Can you work these out from the model? Positions are in its coordinate system, mm. Face numbers are marked on the shaded views. A direction names the side the tool comes from. Give positions to 0.01 mm unless a question says otherwise; leave off trailing zeros. Order: outer loops, then holes, each group sorted by start corner. A loop starts at its lowest first (then second) coordinate and runs counter-clockwise, first axis right, second up.
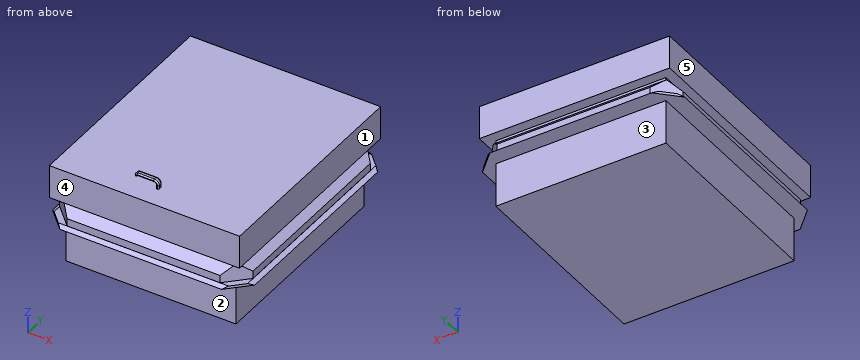
```python
from build123d import *

# Parameters (mm, degrees)
F0_W          = 675
F0_H          = 800
F1_DEPTH      = 270
F2_W          = 755
F2_H          = 880
F3_DEPTH      = 131.76
F5_START      = -175
F4_W          = 802
F4_H          = 926.8378600104
F5_DEPTH      = 10
F6_W          = 767
F6_H          = 892
F7_DEPTH      = 70
F8_SIZE       = 80
F9_SIZE       = 39.99999
F10_SIZE2     = 9.99999
F10_SIZE      = 16.99999
F13_W         = 10
F13_H         = 20
F15_R         = 3.5
F16_T1_DEPTH  = 65
F16_T3_DEPTH  = 3.5995793343
F16_T5_DEPTH  = 13.4709453487
F16_T8_ANGLE  = 90
F16_T10_ANGLE = 90
F16_T12_ANGLE = 90
F16_T14_ANGLE = 90
F16_T16_ANGLE = 90
F16_T18_ANGLE = 90
F16_T20_ANGLE = 90
F16_T22_ANGLE = 90


# Not quite as in the source:
# - a fillet or chamfer that OpenCascade refuses, or shapes differently, is made with other operations: its cross-section is extruded or revolved along the edge and cut away or added
# - a fillet or chamfer is up to 0.001 mm smaller than in the source, because OpenCascade refuses the exact size
# - a feature names something its author has since deleted; it is built from what else it names


with BuildPart() as f1:
    # F0 (on Top) → F1 (new body)
    with BuildSketch(Plane.XY):
        Rectangle(F0_W, F0_H)
    extrude(amount=F1_DEPTH)

    # F2 (on face) → F3 (join)
    with BuildSketch(Plane.XY.offset(270)):
        Rectangle(F2_W, F2_H)
    extrude(amount=F3_DEPTH)

    # F4 (on face) → F5 (join)
    with BuildSketch(Plane(origin=(0, 0, 0), x_dir=(1, 0, 0), z_dir=(0, 0, -1)).offset(F5_START)):
        Rectangle(F4_W, F4_H)
    extrude(amount=-F5_DEPTH)

    # F6 (on face) → F7 (join)
    with BuildSketch(Plane.XY.offset(185)):
        Rectangle(F6_W, F6_H)
    extrude(amount=F7_DEPTH)

    # F8
    f8_edges = [f1.edges().sort_by_distance(p)[0] for p in [
        (383.5, 446, 220),
        (-383.5, 446, 220),
        (-383.5, -446, 220),
        (-401, 463.41893, 180),
        (-401, -463.41893, 180),
        (401, 463.41893, 180),
        (401, -463.41893, 180),
        (383.5, -446, 220),
    ]]
    chamfer(f8_edges, length=F8_SIZE)

    # F9 (size 40 in the source; OpenCascade refuses exactly that, so slightly less here)
    f9_edges = [f1.edges().sort_by_distance(p)[0] for p in [
        (383.5, 0, 255),
        (-383.5, 0, 255),
        (0, 446, 255),
        (0, -446, 255),
    ]]
    chamfer(f9_edges, length=F9_SIZE)

    # F10 (size 17 and 10 in the source; OpenCascade refuses exactly that, so slightly less here)
    f10_edges = [f1.edges().sort_by_distance(p)[0] for p in [
        (-401, 0, 185),
        (0, 463.41893, 185),
        (0, -463.41893, 185),
        (401, 0, 185),
    ]]
    chamfer(f10_edges, length=F10_SIZE, length2=F10_SIZE2)

    # F14: sweep along a path in F12
    with BuildLine(Plane.XZ.offset(350)) as f14_path:
        Line((0, 401.76), (0, 415.2309453487))
        ThreePointArc((0, 415.2309453487), (-4.3933982822, 425.8375470665), (-15, 430.2309453487))
        Line((-15, 430.2309453487), (-80, 430.2309453487))
        ThreePointArc((-80, 430.2309453487), (-83.5355339059, 428.7664792547), (-85, 425.2309453487))
        Line((-85, 425.2309453487), (-85, 421.6313660145))
    # F13 (on face) → F14 (sweep)
    with BuildSketch(Plane.XY.offset(401.76)):
        with Locations((0, -350)):
            Rectangle(F13_W, F13_H)
    sweep(path=f14_path.line)

    # F15
    f15_edges = [f1.edges().sort_by_distance(p)[0] for p in [
        (-90, -350, 421.631366),
        (-85, -360, 421.631366),
        (-80, -350, 421.631366),
        (-85, -340, 421.631366),
    ]]
    fillet(f15_edges, radius=F15_R)

    # F16: fillet of radius 5 on 16 edges, made by hand

    # F16_s2 → F16_t1 (cut)
    with BuildSketch(Plane.YZ.offset(-80)):
        with BuildLine():
            ThreePointArc((-360, 430.2309453487), (-358.5355339059, 433.7664792547), (-355, 435.2309453487))
            Line((-355, 435.2309453487), (-360, 435.2309453487))
            Line((-360, 435.2309453487), (-360, 430.2309453487))
        make_face()
        with BuildLine():
            ThreePointArc((-345, 435.2309453487), (-341.4644660941, 433.7664792547), (-340, 430.2309453487))
            Line((-340, 430.2309453487), (-340, 435.2309453487))
            Line((-340, 435.2309453487), (-345, 435.2309453487))
        make_face()
        with BuildLine():
            ThreePointArc((-360, 430.2309453487), (-358.5355339059, 426.6954114428), (-355, 425.2309453487))
            Line((-355, 425.2309453487), (-360, 425.2309453487))
            Line((-360, 425.2309453487), (-360, 430.2309453487))
        make_face()
        with BuildLine():
            ThreePointArc((-345, 425.2309453487), (-341.4644660941, 426.6954114428), (-340, 430.2309453487))
            Line((-340, 430.2309453487), (-340, 425.2309453487))
            Line((-340, 425.2309453487), (-345, 425.2309453487))
        make_face()
    extrude(amount=F16_T1_DEPTH, mode=Mode.SUBTRACT)

    # F16_s4 → F16_t3 (cut)
    with BuildSketch(Plane.XY.offset(421.6313660145)):
        with BuildLine():
            ThreePointArc((-85, -360), (-88.5355339059, -358.5355339059), (-90, -355))
            Line((-90, -355), (-90, -360))
            Line((-90, -360), (-85, -360))
        make_face()
        with BuildLine():
            ThreePointArc((-90, -345), (-88.5355339059, -341.4644660941), (-85, -340))
            Line((-85, -340), (-90, -340))
            Line((-90, -340), (-90, -345))
        make_face()
    extrude(amount=F16_T3_DEPTH, mode=Mode.SUBTRACT)

    # F16_s6 → F16_t5 (cut)
    with BuildSketch(Plane.XY.offset(401.76)):
        with BuildLine():
            ThreePointArc((0, -360), (3.5355339059, -358.5355339059), (5, -355))
            Line((5, -355), (5, -360))
            Line((5, -360), (0, -360))
        make_face()
        with BuildLine():
            ThreePointArc((0, -360), (-3.5355339059, -358.5355339059), (-5, -355))
            Line((-5, -355), (-5, -360))
            Line((-5, -360), (0, -360))
        make_face()
        with BuildLine():
            ThreePointArc((5, -345), (3.5355339059, -341.4644660941), (0, -340))
            Line((0, -340), (5, -340))
            Line((5, -340), (5, -345))
        make_face()
        with BuildLine():
            ThreePointArc((-5, -345), (-3.5355339059, -341.4644660941), (0, -340))
            Line((0, -340), (-5, -340))
            Line((-5, -340), (-5, -345))
        make_face()
    extrude(amount=F16_T5_DEPTH, mode=Mode.SUBTRACT)

    # F16_s7 → F16_t8 (revolve, cut)
    with BuildSketch(Plane.XZ.offset(345)):
        with BuildLine():
            ThreePointArc((-86.5, 421.6313660145), (-88.9748737342, 422.6564922803), (-90, 425.1313660145))
            Line((-90, 425.1313660145), (-90, 421.6313660145))
            Line((-90, 421.6313660145), (-86.5, 421.6313660145))
        make_face()
    revolve(axis=Axis((-85, -345, 421.6313660145), (0, 0, -1)), revolution_arc=F16_T8_ANGLE, mode=Mode.SUBTRACT)

    # F16_s9 → F16_t10 (revolve, cut)
    with BuildSketch(Plane.YZ.offset(-85)):
        with BuildLine():
            ThreePointArc((-356.5, 421.6313660145), (-358.9748737342, 422.6564922803), (-360, 425.1313660145))
            Line((-360, 425.1313660145), (-360, 421.6313660145))
            Line((-360, 421.6313660145), (-356.5, 421.6313660145))
        make_face()
    revolve(axis=Axis((-85, -355, 421.6313660145), (0, 0, -1)), revolution_arc=F16_T10_ANGLE, mode=Mode.SUBTRACT)

    # F16_s11 → F16_t12 (revolve, cut)
    with BuildSketch(Plane.YZ.offset(-80)):
        with BuildLine():
            ThreePointArc((-360, 430.2309453487), (-358.5355339059, 433.7664792547), (-355, 435.2309453487))
            Line((-355, 435.2309453487), (-360, 435.2309453487))
            Line((-360, 435.2309453487), (-360, 430.2309453487))
        make_face()
    revolve(axis=Axis((-80, -360, 425.2309453487), (0, -1, 0)), revolution_arc=F16_T12_ANGLE, mode=Mode.SUBTRACT)

    # F16_s13 → F16_t14 (revolve, cut)
    with BuildSketch(Plane.XY.offset(415.2309453487)):
        with BuildLine():
            ThreePointArc((0, -360), (3.5355339059, -358.5355339059), (5, -355))
            Line((5, -355), (5, -360))
            Line((5, -360), (0, -360))
        make_face()
    revolve(axis=Axis((-15, -360, 415.2309453487), (0, -1, 0)), revolution_arc=F16_T14_ANGLE, mode=Mode.SUBTRACT)

    # F16_s15 → F16_t16 (revolve, cut)
    with BuildSketch(Plane.XY.offset(415.2309453487)):
        with BuildLine():
            ThreePointArc((0, -360), (-3.5355339059, -358.5355339059), (-5, -355))
            Line((-5, -355), (-5, -360))
            Line((-5, -360), (0, -360))
        make_face()
    revolve(axis=Axis((-15, -360, 415.2309453487), (0, -1, 0)), revolution_arc=F16_T16_ANGLE, mode=Mode.SUBTRACT)

    # F16_s17 → F16_t18 (revolve, cut)
    with BuildSketch(Plane.YZ.offset(-80)):
        with BuildLine():
            ThreePointArc((-345, 435.2309453487), (-341.4644660941, 433.7664792547), (-340, 430.2309453487))
            Line((-340, 430.2309453487), (-340, 435.2309453487))
            Line((-340, 435.2309453487), (-345, 435.2309453487))
        make_face()
    revolve(axis=Axis((-80, -340, 425.2309453487), (0, -1, 0)), revolution_arc=F16_T18_ANGLE, mode=Mode.SUBTRACT)

    # F16_s19 → F16_t20 (revolve, cut)
    with BuildSketch(Plane.XY.offset(415.2309453487)):
        with BuildLine():
            ThreePointArc((5, -345), (3.5355339059, -341.4644660941), (0, -340))
            Line((0, -340), (5, -340))
            Line((5, -340), (5, -345))
        make_face()
    revolve(axis=Axis((-15, -340, 415.2309453487), (0, -1, 0)), revolution_arc=F16_T20_ANGLE, mode=Mode.SUBTRACT)

    # F16_s21 → F16_t22 (revolve, cut)
    with BuildSketch(Plane.XY.offset(415.2309453487)):
        with BuildLine():
            ThreePointArc((-5, -345), (-3.5355339059, -341.4644660941), (0, -340))
            Line((0, -340), (-5, -340))
            Line((-5, -340), (-5, -345))
        make_face()
    revolve(axis=Axis((-15, -340, 415.2309453487), (0, -1, 0)), revolution_arc=F16_T22_ANGLE, mode=Mode.SUBTRACT)


solid = f1.part
```
1) I'm going to push flat-ended pins straight in: pin 1 Ø4 at (x, y) = (-102, -101) entering from +Z; pin 2 Ø1 at (x, z) = (-186.5, 295) entering from -Y; pin 3 Ø24 at (y, z) = (-12.5, 196) entering from +X. Where does each tip first touch, or does it pass through?
2) Suppose I cut it at D-D (z = 349.5). Please give me the cut outline in (x, y).
3) Which directions (+Z, -Z, +X, -X, +Y, -Y) give clear straight access to the entire face, cutting with the end or side of a thin tool? Please do the marked faces 1, 2, 3, 4 and 5.
4) If I drill on line 1 (X direction, y = 223.5, z = 99.5); line 2 (X direction, y = 187, z = 325.5); line 3 (Z direction, x = -56, y = -250), over which ranges is the centre line in solid material (lowest first)?
5) Suppose I cut it at C-C (z = 141). Please give me the cut outline in (x, y), and give its area (3 significant figures).
Results:
1. pin 1: stops at z = 401.76
1. pin 2: stops at y = -440
1. pin 3: stops at x = 385.7
2. outline: (-377.5, -440) - (377.5, -440) - (377.5, 440) - (-377.5, 440) - close
3. face 1: +Z, +X, +Y, -Y
3. face 2: -Z, +X, -X, -Y
3. face 3: -Z, +X, -X, +Y
3. face 4: +Z, +X, -X, -Y
3. face 5: +Z, -X, +Y, -Y
4. line 1: x = -337.5 to 337.5
4. line 2: x = -377.5 to 377.5
4. line 3: z = 0 to 401.76
5. outline: (-337.5, -400) - (337.5, -400) - (337.5, 400) - (-337.5, 400) - close
5. area: 540,000 mm2
